```python
from build123d import *

# Parameters (mm, degrees)
SKETCH5_R           = 4.75
BOSS_EXTRUDE1_DEPTH = 3


with BuildPart() as part:
    # Sketch5 → Boss-Extrude1 (new body)
    with BuildSketch(Plane.XY):
        with Locations((-6.126935789, 33.595569574)):
            Circle(SKETCH5_R)
        with BuildLine():
            Line((-6.156694041, 30.903989601), (-5.607416869, 30.470060358))
            ThreePointArc((-5.607416869, 30.470060358), (-4.946880208, 30.65513141), (-4.341658129, 30.978034198))
            Line((-4.341658129, 30.978034198), (-4.244743599, 31.671292861))
            Line((-4.244743599, 31.671292861), (-3.749736881, 31.729366119))
            Line((-3.749736881, 31.729366119), (-3.810838281, 32.224008185))
            Line((-3.810838281, 32.224008185), (-3.160405947, 32.482731548))
            ThreePointArc((-3.160405947, 32.482731548), (-2.99041385, 33.147308603), (-2.967444827, 33.832897692))
            Line((-2.967444827, 33.832897692), (-3.519367176, 34.263457468))
            Line((-3.519367176, 34.263457468), (-3.322156734, 34.721182491))
            Line((-3.322156734, 34.721182491), (-3.781080029, 34.915588159))
            Line((-3.781080029, 34.915588159), (-3.679924867, 35.608240765))
            ThreePointArc((-3.679924867, 35.608240765), (-4.170469431, 36.087746767), (-4.752722487, 36.450433069))
            Line((-4.752722487, 36.450433069), (-5.401559365, 36.187734182))
            Line((-5.401559365, 36.187734182), (-5.699355642, 36.587385946))
            Line((-5.699355642, 36.587385946), (-6.097177536, 36.287149548))
            Line((-6.097177536, 36.287149548), (-6.646454709, 36.721078791))
            ThreePointArc((-6.646454709, 36.721078791), (-7.30699137, 36.536007739), (-7.912213449, 36.213104951))
            Line((-7.912213449, 36.213104951), (-8.009127978, 35.519846288))
            Line((-8.009127978, 35.519846288), (-8.504134696, 35.46177303))
            Line((-8.504134696, 35.46177303), (-8.443033296, 34.967130964))
            Line((-8.443033296, 34.967130964), (-9.09346563, 34.7084076))
            ThreePointArc((-9.09346563, 34.7084076), (-9.263457727, 34.043830546), (-9.28642675, 33.358241457))
            Line((-9.28642675, 33.358241457), (-8.734504401, 32.92768168))
            Line((-8.734504401, 32.92768168), (-8.931714844, 32.469956658))
            Line((-8.931714844, 32.469956658), (-8.472791548, 32.27555099))
            Line((-8.472791548, 32.27555099), (-8.57394671, 31.582898384))
            ThreePointArc((-8.57394671, 31.582898384), (-8.083402147, 31.103392381), (-7.50114909, 30.74070608))
            Line((-7.50114909, 30.74070608), (-6.852312212, 31.003404967))
            Line((-6.852312212, 31.003404967), (-6.554515936, 30.603753203))
            Line((-6.554515936, 30.603753203), (-6.156694041, 30.903989601))
        make_face(mode=Mode.SUBTRACT)
    extrude(amount=BOSS_EXTRUDE1_DEPTH)


solid = part.part
```
Model file for the job. Use its own axes, mm. A direction names the side the tool comes from. Round coordinates to 2 decimals unless told otherwise and drop trailing zeros. Write each loop counter-clockwise with the first axis right and the second up, starting at its lowest first coordinate (ties: lowest second). Pieces come first, ordered by that corner, then holes. Notation, with made-up numbers: M 19,74 L 72,74 A13 cw 72,94 Z; hole C -4.5,88 d10. An arc over 180 degrees is marked long. Put each result on its own line as item: value.
Item 1: Probe L1, parallel to X at y = 33.5, z = 0.9; L2, parallel to X at y = 36.5, z = 1.25; L3, parallel to X at y = 36.25, z = 0.3. List the from-to ranges inside material, lowest first. Write a range as from..to.
Responses:
L1: -10.88..-9.29, -2.96..-1.38
L2: -9.89..-7.39, -6.37..-5.82, -5.63..-2.37
L3: -10.07..-7.86, -5.45..-5.25, -4.4..-2.19
Item 2: Cut at A-A (y = 35.75). List the corners of the cut face in (x, z).
Responses:
outline: M -10.36,0 L -7.98,0 L -7.98,3 L -10.36,3 Z; M -3.8,0 L -1.89,0 L -1.89,3 L -3.8,3 Z
Item 3: Cut at B-B (x = -4.5). List the corners of the cut face in (y, z), and give its area (3 significant figures).
Responses:
outline: M 29.13,0 L 30.88,0 L 30.88,3 L 29.13,3 Z; M 36.31,0 L 38.06,0 L 38.06,3 L 36.31,3 Z
area: 10.5 mm²
Item 4: Tool access for faces 1 (the flat face through (-6, 30, 3)), 2 (the cylindrical face through (-4.16, 36.08, 1.48)): list every direction of +Z, -Z, +X, -X, +Y, -Y with a clear straight run to the whole face (end or side of a thin tool).
Responses:
face 1: +Z, +X, -X, +Y, -Y
face 2: +Z, -Z
Item 5: Cut at D-D (x = -9.75). List the corners of the cut face in (y, z), and give its area (3 significant figures).
Responses:
outline: M 30.52,0 L 36.67,0 L 36.67,3 L 30.52,3 Z
area: 18.4 mm²
Item 6: Mould opens along X. For faces 3 (the flat face through (-6, 30, 0)), 4 (the cylindrical face through (-3.57, 37.6, 1.48)), 5 (the cylindrical face through (-7.3, 36.54, 1.48)), 6 (the cylindrical face through (-9.262, 34.053, 1.479)) say: +X half, -X half, draft (parallel to the pull), parting line (faces both ways), or undercut.
Responses:
face 3: draft
face 4: parting line
face 5: undercut
face 6: undercut
